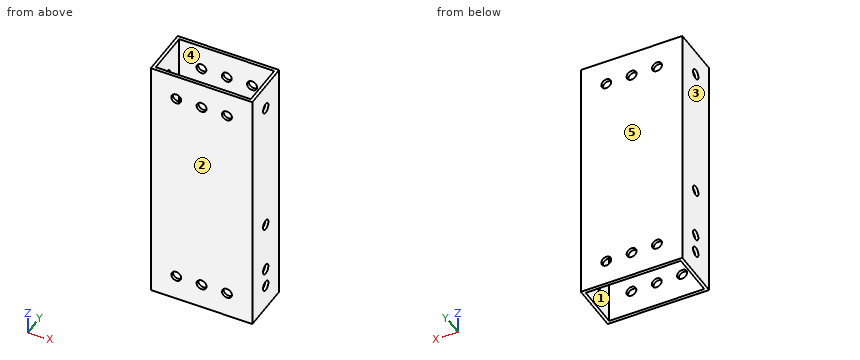
from build123d import *

# Parameters (mm, degrees)
SKETCH1_W           = 50.8
SKETCH1_H           = 25.4
SKETCH1_W_2         = 47.625
SKETCH1_H_2         = 22.225
BOSS_EXTRUDE1_DEPTH = 63.5
SKETCH2_R           = 2.4892
CUT_EXTRUDE1_DEPTH  = 26.4
SKETCH3_R           = 2.4892
CUT_EXTRUDE2_DEPTH  = 51.8
SKETCH5_R           = 2.4892
CUT_EXTRUDE3_DEPTH  = 51.8


with BuildPart() as part:
    # Sketch1 → Boss-Extrude1 (new body, symmetric)
    with BuildSketch(Plane.XY):
        Rectangle(SKETCH1_W, SKETCH1_H)
        Rectangle(SKETCH1_W_2, SKETCH1_H_2, mode=Mode.SUBTRACT)
    extrude(amount=BOSS_EXTRUDE1_DEPTH, both=True)

    # Sketch2 → Cut-Extrude1 (cut, through all)
    with BuildSketch(Plane(origin=(0, 12.7, 0), x_dir=(1, 0, 0), z_dir=(0, 1, 0))):
        with Locations((-12.7, 50.8)):
            Circle(SKETCH2_R)
        with Locations((0, 50.8)):
            Circle(SKETCH2_R)
        with Locations((12.7, 50.8)):
            Circle(SKETCH2_R)
        with Locations((12.7, -50.8)):
            Circle(SKETCH2_R)
        with Locations((0, -50.8)):
            Circle(SKETCH2_R)
        with Locations((-12.7, -50.8)):
            Circle(SKETCH2_R)
    extrude(amount=-CUT_EXTRUDE1_DEPTH, mode=Mode.SUBTRACT)

    # Sketch3 → Cut-Extrude2 (cut, through all)
    with BuildSketch(Plane.ZY.offset(25.4)):
        with Locations((-50.8, 0)):
            Circle(SKETCH3_R)
        with Locations((50.8, 0)):
            Circle(SKETCH3_R)
    extrude(amount=-CUT_EXTRUDE2_DEPTH, mode=Mode.SUBTRACT)

    # Sketch5 → Cut-Extrude3 (cut, through all)
    with BuildSketch(Plane(origin=(25.4, 0, 0), x_dir=(0, 0, -1), z_dir=(1, 0, 0))):
        with Locations((41.275, 0)):
            Circle(SKETCH5_R)
        with Locations((15.875, 0)):
            Circle(SKETCH5_R)
    extrude(amount=-CUT_EXTRUDE3_DEPTH, mode=Mode.SUBTRACT)


solid = part.part
Here's how the part is built. I have some questions about the finished solid (model axes, mm). Face numbers are marked on the shaded views. A direction names the side the tool comes from. Coordinates: 2 decimals unless noted, no trailing zeros. Order: outer loops, then holes, each group sorted by start corner. A loop starts at its lowest first (then second) coordinate and runs counter-clockwise, first axis right, second up. Notation, with made-up numbers: (-14.5, -31.5) - (25.5, -31.5) arc R5 cw to (25.5, -22.5) - close; hole circle Ø7 at (-31.5, 69.5). An arc over 180 degrees is marked (long way). Use CSV: the item, a comma, the result in double quotes. Start each with the question number.
1. Suppose I cut it at A-A on y = 8.5. List the corners of the cut face in (x, z) for me.
2. Please list where these lines run through material, in increasing order: line 1 (X direction, y = -11.45, z = -50.8); line 2 (Z direction, x = -12.7, y = -11.5); line 3 (Y direction, x = -22, z = -15). Write a range as from..to.
3. For the marked faces 4 and 5, which set-ups out of +Z, -Z, +X, -X, +Y, -Y let a thin tool reach every point of the face, with its end or its side?
4. If we mould it in two halves opening along X, with no side actions, what happens to the marked faces 1, 2 and 3? For each: +X half, -X half, draft (parallel to the pull), parting line (faces both ways), or undercut.
5. Suppose I cut it at C-C on z = 24. List the corners of the cut face in (x, y) for me.
6. I'm going to push flat-ended pins straight in: pin 1 (4 mm diameter, centred on x = 12.7, z = 50.8, fed in from -Y); pin 2 (10 mm diameter, centred on x = 19.5, y = 9, fed in from -Z). Where does each tip first touch, or does it pass through?
7. Suppose I cut it at D-D on x = -7. List the corners of the cut face in (y, z) for me, then the cut area to 3 significant figures.
8. Suppose I cut it at B-B on x = -12.7. List the corners of the cut face in (y, z) for me.
Output:
1,outline,"(-25.4, -63.5) - (-23.81, -63.5) - (-23.81, 63.5) - (-25.4, 63.5) - close; (23.81, -63.5) - (25.4, -63.5) - (25.4, 63.5) - (23.81, 63.5) - close"
2,line 1,"x = -25.4..-15.19, -10.21..-2.49, 2.49..10.21, 15.19..25.4"
2,line 2,"z = -63.5..-53.29, -48.31..48.31, 53.29..63.5"
2,line 3,"y = -12.7..-11.11, 11.11..12.7"
3,face 4,"+Z, -Z"
3,face 5,"+Z, -Z, +X, -X, +Y"
4,face 1,"undercut"
4,face 2,"draft"
4,face 3,"-X half"
5,outline,"(-25.4, -12.7) - (25.4, -12.7) - (25.4, 12.7) - (-25.4, 12.7) - close; hole (-23.81, -11.11) - (23.81, -11.11) - (23.81, 11.11) - (-23.81, 11.11) - close"
6,pin 1,"passes through"
6,pin 2,"stops at z = -63.5"
7,outline,"(-12.7, -63.5) - (-11.11, -63.5) - (-11.11, 63.5) - (-12.7, 63.5) - close; (11.11, -63.5) - (12.7, -63.5) - (12.7, 63.5) - (11.11, 63.5) - close"
7,area,"403 mm2"
8,outline,"(-12.7, -63.5) - (-11.11, -63.5) - (-11.11, -53.29) - (-12.7, -53.29) - close; (-12.7, -48.31) - (-11.11, -48.31) - (-11.11, 48.31) - (-12.7, 48.31) - close; (-12.7, 53.29) - (-11.11, 53.29) - (-11.11, 63.5) - (-12.7, 63.5) - close; (11.11, -63.5) - (12.7, -63.5) - (12.7, -53.29) - (11.11, -53.29) - close; (11.11, -48.31) - (12.7, -48.31) - (12.7, 48.31) - (11.11, 48.31) - close; (11.11, 53.29) - (12.7, 53.29) - (12.7, 63.5) - (11.11, 63.5) - close"
